The model under review builds one solid part; all positions refer to its coordinate system, in mm. Face numbers are marked on the shaded views. Give positions to 0.01 mm unless a question says otherwise; leave off trailing zeros. Order: outer loops, then holes, each group sorted by start corner. A loop starts at its lowest first (then second) coordinate and runs counter-clockwise, first axis right, second up. Notation, with made-up numbers: M 26,-27 L 73,-27 A28 ccw 73,-2 Z; hole C -11,9 d1. An arc over 180 degrees is marked long. One line per question, with ' | ' between items. Start each with the question number.
1. Wall thickness on L1, parallel to Y at x = 0, z = 1; L2, parallel to Y at x = -0.5, z = -0.6; L3, parallel to X at y = 6, z = 0.55: over which ranges is each line inside the solid? List them lowest first.
2. Insertion check: P1, Ø4, axis at x = -0.5, y = 6.5, coming from the -Z side; P2, Ø2.5, axis at x = 0, y = 6, coming from the -Z side; P3, Ø1.5, axis at x = -2, z = 0, coming from the +Y side. Each pin has a flat end and moves straight along its axis. Give the tip position at first contact, or say it passes through.
3. We need section D-D on y = -6.25. Write out the cut boundary in (x, z), then the cut area to 3 significant figures.
4. We need section A-A on z = 0.6. Count the separate pieces of the cut face and the enclosed holes in it, then the cut area to 3 significant figures.
5. We need section B-B on y = 6.75. Write out the cut boundary in (x, z), then the cut area to 3 significant figures.
6. We need section C-C on x = 1. Write out the cut boundary in (y, z), then the cut area to 3 significant figures.
7. The part is to be moulded in two halves that separate along Y. For the marked faces 1, 2 and 3, say which applies: +Y half, -Y half, draft (parallel to the pull), parting line (faces both ways), or undercut.
Solid Edge part; units mm, degrees
sketch "Sketch1" plane through (0, 0, 0) normal (0, -1, 0) x (1, 0, 0)
  line L0 (-3.5, -1.5) -> (3.5, -1.5)
  line L1 (3.5, -1.5) -> (3.5, 1.5)
  line L2 (3.5, 1.5) -> (-3.5, 1.5)
  line L3 (-3.5, 1.5) -> (-3.5, -1.5)
  dimension "D1" = 3.5
  dimension "D2" = 3.5
extrude "Protrusion1" add sketch "Sketch1" along normal mid plane 18
sketch "Sketch2" plane through (0, 0, 1.5) normal (0, 0, 1) x (0, 1, 0)
  circle A0 centre (6, 0) radius 1.5
  circle A1 centre (-6, 0) radius 1.5
extrude "Cutout1" cut sketch "Sketch2" against normal blind 6.4951
fillet "Round_3" radius 3.5 4 edges at (-3.5, -9, 0) (3.5, -9, 0) (3.5, 9, 0) (-3.5, 9, 0)
properties material "Aluminum, 6061-T6"
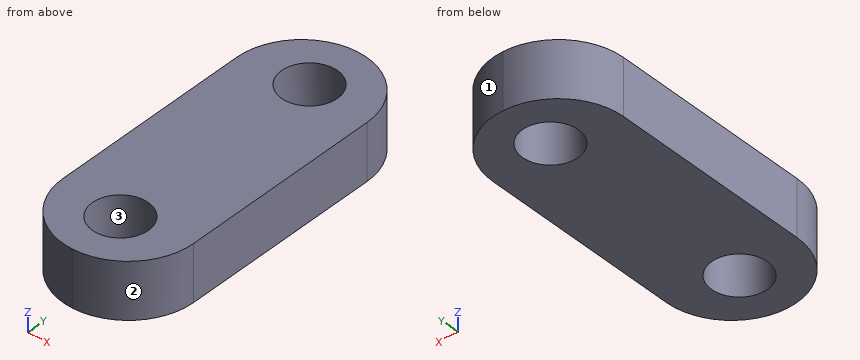
Entries:
1) L1: y = -9 to -7.5, -4.5 to 4.5, 7.5 to 9 | L2: y = -8.96 to -7.41, -4.59 to 4.59, 7.41 to 8.96 | L3: x = -3.46 to -1.5, 1.5 to 3.46
2) P1: stops at z = -1.5 | P2: passes through | P3: stops at y = 8.77
3) outline: M -3.42,-1.5 L -1.48,-1.5 L -1.48,1.5 L -3.42,1.5 Z; M 1.48,-1.5 L 3.42,-1.5 L 3.42,1.5 L 1.48,1.5 Z | area: 11.6 mm^2
4) separate pieces: 1 | enclosed holes: 2 | area: 101 mm^2
5) outline: M -3.27,-1.5 L -1.3,-1.5 L -1.3,1.5 L -3.27,1.5 Z; M 1.3,-1.5 L 3.27,-1.5 L 3.27,1.5 L 1.3,1.5 Z | area: 11.8 mm^2
6) outline: M -8.85,-1.5 L -7.12,-1.5 L -7.12,1.5 L -8.85,1.5 Z; M -4.88,-1.5 L 4.88,-1.5 L 4.88,1.5 L -4.88,1.5 Z; M 7.12,-1.5 L 8.85,-1.5 L 8.85,1.5 L 7.12,1.5 Z | area: 39.7 mm^2
7) face 1: +Y half | face 2: -Y half | face 3: undercut
